Verification items for the finished model (mm, model axes). Round coordinates to 2 decimals unless told otherwise and drop trailing zeros. Write each loop counter-clockwise with the first axis right and the second up, starting at its lowest first coordinate (ties: lowest second). Pieces come first, ordered by that corner, then holes. Notation, with made-up numbers: (-35, 50) - (-31, 50) arc R12 ccw to (-31, 63) - close; hole circle Ø4 at (17.5, 67). An arc over 180 degrees is marked (long way). Answer as a JSON object with one key per item and string values.
```python
from build123d import *

# Parameters (mm, degrees)
F0_W     = 508
F0_H     = 1016
F1_DEPTH = 101.6
F2_R     = 25.4
F2_R_2   = 39.6875
F3_DEPTH = 101.601
F4_R     = 12.7


with BuildPart() as f1:
    # F0 (on Top) → F1 (new body)
    with BuildSketch(Plane.XY):
        Rectangle(F0_W, F0_H)
    extrude(amount=F1_DEPTH)

    # F2 (on face) → F3 (cut, through all)
    with BuildSketch(Plane.XY.offset(101.6)):
        with Locations((-120.65, -355.6)):
            Circle(F2_R)
        with Locations((120.65, -355.6)):
            Circle(F2_R)
        with Locations((0, 63.5)):
            Circle(F2_R_2)
        with Locations((0, 381)):
            Circle(F2_R_2)
    extrude(amount=-F3_DEPTH, mode=Mode.SUBTRACT)

    # F4
    f4_edges = [f1.edges().sort_by_distance(p)[0] for p in [
        (-254, -508, 50.8),
        (254, -508, 50.8),
        (254, 508, 50.8),
        (-254, 508, 50.8),
    ]]
    fillet(f4_edges, radius=F4_R)


solid = f1.part
```
1. Mould release check, pull along Y, two halves, no side actions. Record for faces 1 (the face through (-3, 508, 50)), 2 (the face through (-123.957, -330.416, 51.511)), 3 (the face through (-254, -7, 50)): released by +Y, released by -Y, zero draft, split by the parting line, or undercut.
Completed:
{"face 1": "released by +Y", "face 2": "undercut", "face 3": "zero draft"}
2. Cross-section at B-B (y = 381). Record the boundary of the cut face in (x, z).
Completed:
{"outline": "(-254, 0) - (-39.69, 0) - (-39.69, 101.6) - (-254, 101.6) - close; (39.69, 0) - (254, 0) - (254, 101.6) - (39.69, 101.6) - close"}
3. Cross-section at C-C (x = 0). Record the boundary of the cut face in (y, z), plus the area to 3 significant figures.
Completed:
{"outline": "(-508, 0) - (23.81, 0) - (23.81, 101.6) - (-508, 101.6) - close; (103.19, 0) - (341.31, 0) - (341.31, 101.6) - (103.19, 101.6) - close; (420.69, 0) - (508, 0) - (508, 101.6) - (420.69, 101.6) - close", "area": "87,100 mm^2"}
4. Cross-section at A-A (z = 50). Count the separate pieces of the cut face and the enclosed holes in it, plus the area to 3 significant figures.
Completed:
{"separate pieces": "1", "enclosed holes": "4", "area": "502,000 mm^2"}
5. Cross-section at D-D (x = 120.65). Record the boundary of the cut face in (y, z).
Completed:
{"outline": "(-508, 0) - (-381, 0) - (-381, 101.6) - (-508, 101.6) - close; (-330.2, 0) - (508, 0) - (508, 101.6) - (-330.2, 101.6) - close"}
6. Material ranges on probe 1 along Y at (x, z) = (0, 62.5); probe 2 along Y at (x, z) = (120, 80); probe 3 along X at (y, z) = (-355, 55), recorded low to high. Write a range as from..to.
Completed:
{"probe 1": "y = -508..23.81, 103.19..341.31, 420.69..508", "probe 2": "y = -508..-380.99, -330.21..508", "probe 3": "x = -254..-146.04, -95.26..95.26, 146.04..254"}
